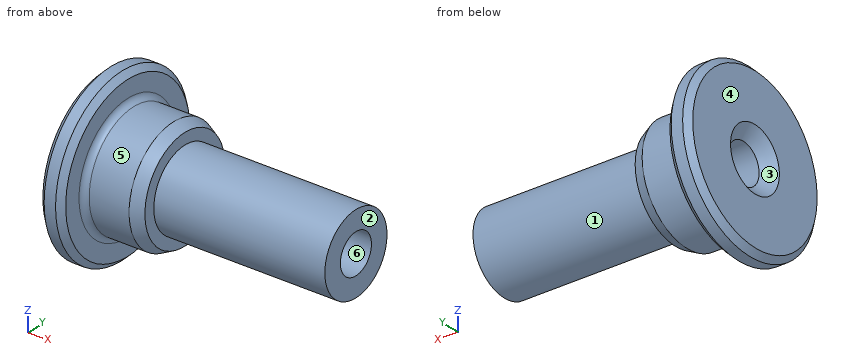
```python
from build123d import *

# Parameters (mm, degrees)
FILLET1_R          = 0.5
CHAMFER1_SIZE      = 0.5
SKETCH2_R          = 1.75
CUT_EXTRUDE1_DEPTH = 23
CHAMFER2_SIZE      = 1


with BuildPart() as part:
    # Sketch1 → Revolve1 (revolve)
    with BuildSketch(Plane.XY):
        Polygon((0, 0), (0, 7.5), (2, 7.5), (2, 5), (6, 5), (7, 4.5), (7, 3.5), (22, 3.5), (22, 0), align=None)
    revolve(axis=Axis((0, 0, 0), (1, 0, 0)))

    # Fillet1
    fillet1_edges = [part.edges().sort_by_distance(p)[0] for p in [
        (2, -5, 0),
    ]]
    fillet(fillet1_edges, radius=FILLET1_R)

    # Chamfer1
    chamfer1_edges = [part.edges().sort_by_distance(p)[0] for p in [
        (2, -7.5, 0),
        (0, -7.5, 0),
    ]]
    chamfer(chamfer1_edges, length=CHAMFER1_SIZE)

    # Sketch2 → Cut-Extrude1 (cut, through all)
    with BuildSketch(Plane(origin=(22, 0, 0), x_dir=(0, 0, -1), z_dir=(1, 0, 0))):
        Circle(SKETCH2_R)
    extrude(amount=-CUT_EXTRUDE1_DEPTH, mode=Mode.SUBTRACT)

    # Chamfer2
    chamfer2_edges = [part.edges().sort_by_distance(p)[0] for p in [
        (0, 0, 1.75),
    ]]
    chamfer(chamfer2_edges, length=CHAMFER2_SIZE)


solid = part.part
```
The listing builds one solid part. Answer for the finished solid, in the listing's coordinates (mm). Face numbers are marked on the shaded views. A direction names the side the tool comes from. Round coordinates to 2 decimals unless told otherwise and drop trailing zeros. Order: outer loops, then holes, each group sorted by start corner. A loop starts at its lowest first (then second) coordinate and runs counter-clockwise, first axis right, second up. Notation, with made-up numbers: (41, 51.5) -> (85, 51.5) arc R14 ccw to (85, 55.5) -> close; hole circle Ø1 at (-20.5, -28). An arc over 180 degrees is marked (long way). Answer as CSV lines item,"result". Start each with the question number.
(1) The part is cut by section C-C (x = 5.75). Determine the outline of the cut face in (y, z).
(2) For a pull along Z with two mould halves and no side action, classify the marked faces 3, 4, 5 and 6 as +Z half, -Z half, draft (parallel to the pull), parting line (faces both ways), or undercut.
(3) The part is cut by section A-A (y = 0). Determine the outline of the cut face in (x, z).
(4) Find the intervals of material crossed by probe 1 along X at (y, z) = (-4, 5); probe 2 along Y at (x, z) = (3.25, -1.25); probe 3 along Z at (x, y) = (2.25, 0.75), in increasing order. Write a range as from..to.
(5) Flat-ended cylindrical pins translate along their axes: pin 1 Ø5 at (x, z) = (6.5, -4.5) entering from -Y; pin 2 Ø8 at (x, z) = (15.5, -2.5) entering from +Y; pin 3 Ø8 at (x, z) = (5.5, -5.5) entering from -Y. Find the tip coordinate at first contact, or state that the pin passes through.
(6) A tool of negligible diameter and unlimited length cuts with its end or side. For the marked faces 1 and 2, from which of +Z, -Z, +X, -X, +Y, -Y can it reach the whole face along a straight path? Write none if from no direction.
(7) The part is cut by section B-B (x = 10). Determine the outline of the cut face in (y, z).
Evaluation:
1,outline,"circle Ø10 at (0, 0); hole circle Ø3.5 at (0, 0)"
2,face 3,"undercut"
2,face 4,"draft"
2,face 5,"parting line"
2,face 6,"undercut"
3,outline,"(0, -7) -> (0.5, -7.5) -> (1.5, -7.5) -> (2, -7) -> (2, -5.5) arc R0.5 cw to (2.5, -5) -> (6, -5) -> (7, -4.5) -> (7, -3.5) -> (22, -3.5) -> (22, -1.75) -> (1, -1.75) -> (0, -2.75) -> close; (0, 2.75) -> (1, 1.75) -> (22, 1.75) -> (22, 3.5) -> (7, 3.5) -> (7, 4.5) -> (6, 5) -> (2.5, 5) arc R0.5 cw to (2, 5.5) -> (2, 7) -> (1.5, 7.5) -> (0.5, 7.5) -> (0, 7) -> close"
4,probe 1,"0..2"
4,probe 2,"-4.84..-1.22, 1.22..4.84"
4,probe 3,"-5.01..-1.58, 1.58..5.01"
5,pin 1,"y = -4.56"
5,pin 2,"y = 3.5"
5,pin 3,"y = -6.03"
6,face 1,"+X"
6,face 2,"+Z, -Z, +X, +Y, -Y"
7,outline,"circle Ø7 at (0, 0); hole circle Ø3.5 at (0, 0)"
